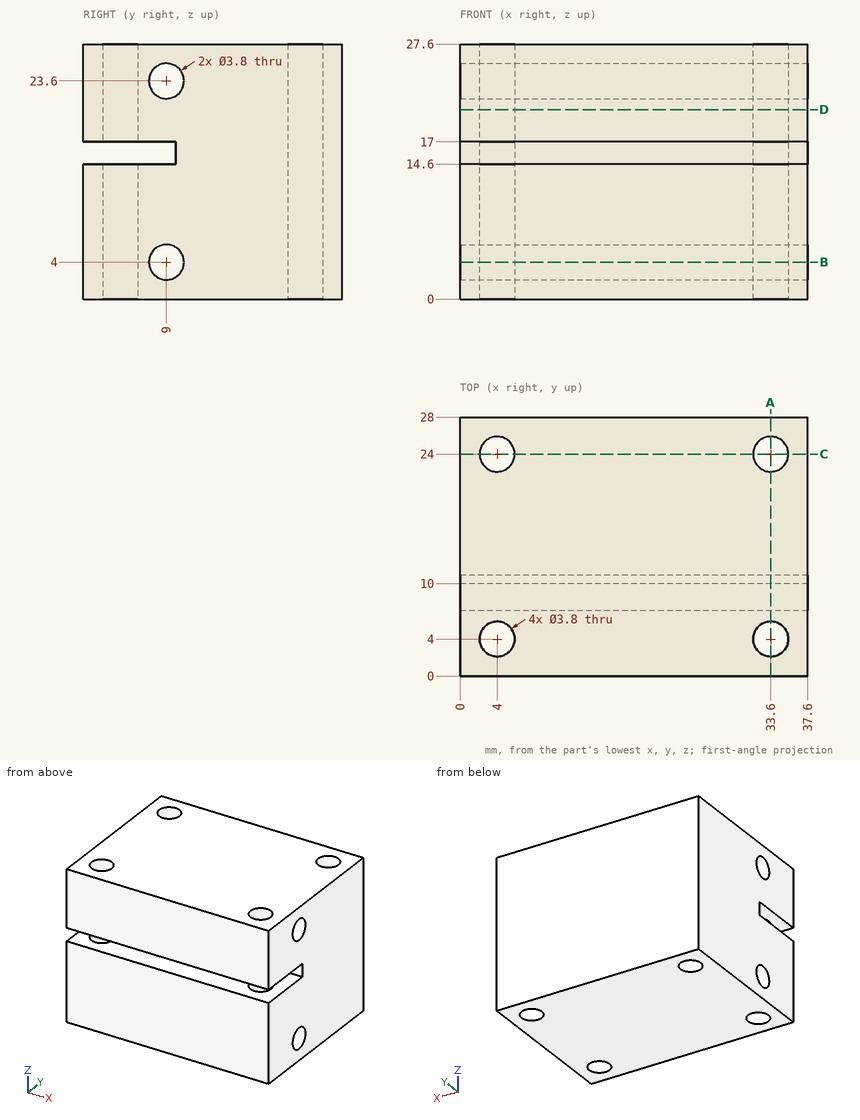
Source: three-view drawing plus pictorial views. Frame: mm from the lowest corner of the part. Round coordinates to 2 decimals unless told otherwise and drop trailing zeros. Write each loop counter-clockwise with the first axis right and the second up, starting at its lowest first coordinate (ties: lowest second). Pieces come first, ordered by that corner, then holes. Notation, with made-up numbers: M -18,32 L -4,32 A25 ccw -4,70 Z; hole C 18,47.5 d6. An arc over 180 degrees is marked long. Use CSV: the item, a comma, the result in double quotes. Start each with the question number.
Q1. Cut plane B-B on z = 4. Output: boundary loops of the cut face in (x, y).
Q2. Line query: line 1 (X direction, y = 4, z = 22); line 2 (Z direction, x = 16, y = 9); line 3 (Y direction, x = 34.5, z = 12.25). Output: solid intervals per line, ascending. Write a range as from..to.
Q3. Cut plane D-D on z = 20.5. Output: boundary loops of the cut face in (x, y).
Q4. Cut plane A-A on x = 33.6. Output: boundary loops of the cut face in (y, z).
Q5. Cut plane C-C on y = 24. Output: boundary loops of the cut face in (x, z).
Results found:
1,outline,"M 0,0 L 37.6,0 L 37.6,7.1 L 0,7.1 Z; M 0,10.9 L 37.6,10.9 L 37.6,28 L 0,28 Z; hole C 4,4 d3.8; hole C 4,24 d3.8; hole C 33.6,4 d3.8; hole C 33.6,24 d3.8"
2,line 1,"0..2.1, 5.9..31.7, 35.5..37.6"
2,line 2,"0..2.1, 5.9..14.6, 17..21.7, 25.5..27.6"
2,line 3,"0..2.33, 5.67..22.33, 25.67..28"
3,outline,"M 0,0 L 37.6,0 L 37.6,28 L 0,28 Z; hole C 4,4 d3.8; hole C 4,24 d3.8; hole C 33.6,4 d3.8; hole C 33.6,24 d3.8"
4,outline,"M 0,0 L 2.1,0 L 2.1,14.6 L 0,14.6 Z; M 0,17 L 2.1,17 L 2.1,27.6 L 0,27.6 Z; M 5.9,0 L 22.1,0 L 22.1,27.6 L 5.9,27.6 L 5.9,17 L 10,17 L 10,14.6 L 5.9,14.6 Z; M 25.9,0 L 28,0 L 28,27.6 L 25.9,27.6 Z; hole C 9,4 d3.8; hole C 9,23.6 d3.8"
5,outline,"M 0,0 L 2.1,0 L 2.1,27.6 L 0,27.6 Z; M 5.9,0 L 31.7,0 L 31.7,27.6 L 5.9,27.6 Z; M 35.5,0 L 37.6,0 L 37.6,27.6 L 35.5,27.6 Z"
